from build123d import *

# Parameters (mm, degrees)
BASE_FLANGE1_DEPTH              = 6
SKETCH2_W                       = 1968.518691842
SKETCH2_H                       = 782.123286761
CUT_EXTRUDE1_DEPTH              = 10
SKETCH3_R                       = 3.5
CUT_EXTRUDE2_DEPTH              = 10
CIRPATTERN4_COUNT               = 7
CIRPATTERN4_ANGLE               = 63
CIRPATTERN4_THE_OTHER_WAY_COUNT = 7
CIRPATTERN4_THE_OTHER_WAY_ANGLE = 63


# Sheet-metal steps are written as plain solids
with BuildPart() as part:
    # Sketch1 → Base-Flange1 (new body)
    with BuildSketch(Plane.XY):
        with BuildLine():
            Line((859.985464993, -5), (-859.985464993, -5))
            ThreePointArc((-859.985464993, -5), (0, -860), (859.985464993, -5))
        make_face()
    extrude(amount=-BASE_FLANGE1_DEPTH)

    # Sketch2 → Cut-Extrude1 (cut)
    with BuildSketch(Plane.XY):
        with Locations((10.387961435, 27.061643381)):
            Rectangle(SKETCH2_W, SKETCH2_H)
    extrude(amount=-CUT_EXTRUDE1_DEPTH, mode=Mode.SUBTRACT)

    # Sketch3 → Cut-Extrude2 (cut)
    with BuildSketch(Plane(origin=(0, 0, -6), x_dir=(-1, 0, 0), z_dir=(0, 0, -1))):
        with Locations((0, -820)):
            Circle(SKETCH3_R)
    cut_extrude2 = extrude(amount=-CUT_EXTRUDE2_DEPTH, mode=Mode.SUBTRACT)

    # CirPattern4: Cut-Extrude2 ×7 about axis
    cirpattern4_axis = Axis((0, 0, 0), (0, 0, 1))
    for i in range(1, CIRPATTERN4_COUNT):
        add(cut_extrude2.rotate(cirpattern4_axis, i * CIRPATTERN4_ANGLE / (CIRPATTERN4_COUNT - 1)), mode=Mode.SUBTRACT)

    # CirPattern4 the other way: Cut-Extrude2 ×7 about axis
    cirpattern4_the_other_way_axis = Axis((0, 0, 0), (0, 0, -1))
    for i in range(1, CIRPATTERN4_THE_OTHER_WAY_COUNT):
        add(cut_extrude2.rotate(cirpattern4_the_other_way_axis, i * CIRPATTERN4_THE_OTHER_WAY_ANGLE / (CIRPATTERN4_THE_OTHER_WAY_COUNT - 1)), mode=Mode.SUBTRACT)


solid = part.part
Can you work these out from the model? Positions are in its coordinate system, mm. Coordinates: 2 decimals unless noted, no trailing zeros. Loops run counter-clockwise (first coordinate to the right, second up) from the corner with the lowest first, then second, coordinate; pieces in that order, holes last. Notation, with made-up numbers: (56, 38) - (72, 38) arc R14 cw to (72, 65) - close; hole circle Ø2 at (2.25, 49.5). An arc over 180 degrees is marked (long way). Answer as a JSON object with one key per item and string values. Group by question number.
Item 1: If I drill on L1, parallel to Y at x = -147.5, z = -4.5; L2, parallel to X at y = -599, z = -3.25; L3, parallel to Y at x = -221.5, z = -3, over which ranges is the centre line in solid material (lowest first)? Write a range as from..to.
Item 2: For pin 1 (6.5 mm diameter, centred on x = -293.86, y = -765.54, fed in from +Z) (3 decimals); pin 2 (1 mm diameter, centred on x = -378, z = -3, fed in from -Y), each with a flat end and sliding along its axis, tell me the tip position at first contact or that it passes through.
Item 3: If we section it at C-C (x = -224): List the corners of the cut face in (y, z) for me.
Item 4: If we section it at B-B (y = -653.5): List the corners of the cut face in (x, z) for me, plus the area to 3 significant figures.
Item 5: If we section it at A-A (z = -2.85): State how many separate pieces and enclosed holes the cut face has, plus the area to 3 significant figures.
Returned:
{
 "1": {"L1": "y = -847.26..-809.19, -803.35..-364", "L2": "x = -617.09..617.09", "L3": "y = -830.99..-364"},
 "2": {"pin 1": "passes through", "pin 2": "stops at y = -772.72"},
 "3": {"outline": "(-830.32, -6) - (-364, -6) - (-364, 0) - (-830.32, 0) - close"},
 "4": {"outline": "(-559.05, -6) - (559.05, -6) - (559.05, 0) - (-559.05, 0) - close", "area": "6,710 mm²"},
 "5": {"separate pieces": "1", "enclosed holes": "13", "area": "554,000 mm²"}
}
